Part model, mm, in its own coordinate system. A direction names the side the tool comes from. Give positions to 0.01 mm unless a question says otherwise; leave off trailing zeros. Order: outer loops, then holes, each group sorted by start corner. A loop starts at its lowest first (then second) coordinate and runs counter-clockwise, first axis right, second up. Notation, with made-up numbers: M 14.5,46.25 L 31.5,46.25 A14 ccw 31.5,53.25 Z; hole C -6,81 d2. An arc over 180 degrees is marked long. Answer as a JSON object with one key per item and string values.
from build123d import *

# Parameters (mm, degrees)
SKETCH1_W           = 30
SKETCH1_H           = 20
SKETCH1_H_2         = 2.5
SKETCH1_W_2         = 16
SKETCH1_W_3         = 7
SKETCH1_H_3         = 10.6
BOSS_EXTRUDE1_DEPTH = 6
SKETCH1_3_W         = 7
SKETCH1_3_H         = 2.5
SKETCH1_3_W_2       = 16
SKETCH1_3_W_3       = 30
BOSS_EXTRUDE2_DEPTH = 12
SKETCH3_R           = 1.5
CUT_EXTRUDE2_DEPTH  = 15
CUT_EXTRUDE1_DEPTH  = 38.976966704


with BuildPart() as part:
    # Sketch1 → Boss-Extrude1 (new body)
    with BuildSketch(Plane(origin=(0, 0, 0), x_dir=(1, 0, 0), z_dir=(0, 1, 0))):
        with Locations((-15, -10)):
            Rectangle(SKETCH1_W, SKETCH1_H)
        with Locations((-15, -21.25)):
            Rectangle(SKETCH1_W, SKETCH1_H_2)
        with Locations((-15, 1.25)):
            Rectangle(SKETCH1_W_2, SKETCH1_H_2)
        with Locations((-3.5, 1.25)):
            Rectangle(SKETCH1_W_3, SKETCH1_H_2)
        with Locations((-3.5, 7.8)):
            Rectangle(SKETCH1_W_3, SKETCH1_H_3)
        with Locations((-3.5, 14.35)):
            Rectangle(SKETCH1_W_3, SKETCH1_H_2)
        with Locations((-15, 14.35)):
            Rectangle(SKETCH1_W_2, SKETCH1_H_2)
        with Locations((-26.5, 14.35)):
            Rectangle(SKETCH1_W_3, SKETCH1_H_2)
        with Locations((-26.5, 7.8)):
            Rectangle(SKETCH1_W_3, SKETCH1_H_3)
        with Locations((-26.5, 1.25)):
            Rectangle(SKETCH1_W_3, SKETCH1_H_2)
    extrude(amount=BOSS_EXTRUDE1_DEPTH)

    # Sketch1_3 → Boss-Extrude2 (add)
    with BuildSketch(Plane(origin=(0, 0, 0), x_dir=(1, 0, 0), z_dir=(0, 1, 0))):
        with Locations((-3.5, 1.25)):
            Rectangle(SKETCH1_3_W, SKETCH1_3_H)
        with Locations((-15, 1.25)):
            Rectangle(SKETCH1_3_W_2, SKETCH1_3_H)
        with Locations((-15, -21.25)):
            Rectangle(SKETCH1_3_W_3, SKETCH1_3_H)
        with Locations((-26.5, 1.25)):
            Rectangle(SKETCH1_3_W, SKETCH1_3_H)
    extrude(amount=BOSS_EXTRUDE2_DEPTH)

    # Sketch3 → Cut-Extrude2 (cut)
    with BuildSketch(Plane(origin=(0, 0, -15.6), x_dir=(-1, 0, 0), z_dir=(0, 0, -1))):
        with Locations((15, 3)):
            Circle(SKETCH3_R)
    extrude(amount=-CUT_EXTRUDE2_DEPTH, mode=Mode.SUBTRACT)

    # Sketch2 → Cut-Extrude1 (cut, through all)
    with BuildSketch(Plane(origin=(0, 6, 0), x_dir=(1, 0, 0), z_dir=(0, 1, 0))):
        with BuildLine():
            ThreePointArc((-13, -10), (-15, -8), (-17, -10))
            Line((-17, -10), (-13, -10))
        make_face()
        with BuildLine():
            Line((-13, -10), (-17, -10))
            ThreePointArc((-17, -10), (-15, -12), (-13, -10))
        make_face()
    extrude(amount=-CUT_EXTRUDE1_DEPTH, mode=Mode.SUBTRACT)


solid = part.part
1. Probe line 1 along Z through (x, y) = (-20.5, 4); line 2 along Z through (x, y) = (-21.25, 9.5); line 3 along Z through (x, y) = (-15, 1.3). List the from-to ranges inside material, lowest first.
Worked answers:
{"line 1": "z = -15.6 to -13.1, -2.5 to 22.5", "line 2": "z = -2.5 to 0, 20 to 22.5", "line 3": "z = -15.6 to -13.1, -2.5 to 8, 12 to 22.5"}
2. Cut at C-C on z = 10. Give the cut face in (x, y).
Worked answers:
{"outline": "M -30,0 L -17,0 L -17,6 L -30,6 Z; M -13,0 L 0,0 L 0,6 L -13,6 Z"}
3. Cut at A-A on x = -20. Give the cut face in (y, z).
Worked answers:
{"outline": "M 0,-15.6 L 6,-15.6 L 6,-13.1 L 0,-13.1 Z; M 0,-2.5 L 12,-2.5 L 12,0 L 6,0 L 6,20 L 12,20 L 12,22.5 L 0,22.5 Z"}
4. Cut at B-B on y = 10. Give the cut face in (x, z).
Worked answers:
{"outline": "M -30,-2.5 L 0,-2.5 L 0,0 L -30,0 Z; M -30,20 L 0,20 L 0,22.5 L -30,22.5 Z"}
5. Two-plate mould, pull along Z, no slides. Class faces 1 (the cylindrical face through (-13.526, 3.042, 11.352)), 2 (the flat face through (-23, 3, -8)), 3 (the flat face through (-15, 6, 22.5)), 4 (the flat face through (-30, 5, 3)): +Z half, -Z half, draft (parallel to the pull), parting line (faces both ways), or undercut.
Worked answers:
{"face 1": "undercut", "face 2": "undercut", "face 3": "+Z half", "face 4": "draft"}
6. Which spindle directions (+Z, -Z, +X, -X, +Y, -Y) get a long thin tool onto all of the face, cutting with end or side? Do faces 5 (the flat face through (-7, 3, -8)), 6 (the flat face through (-15.2, 6, 7.6)), 7 (the flat face through (-15, 7, -2.5)), 8 (the flat face through (-15, 6, -14)), 9 (the cylindrical face through (-13.5, 3.07, -14.37)). Say none if no direction does.
Worked answers:
{"face 5": "+Y, -Y", "face 6": "+X, -X, +Y", "face 7": "+Y", "face 8": "-Z, +X, -X, +Y", "face 9": "-Z"}
7. Pin check, flat tips, straight feed: P1, Ø0.9, axis at x = -15.5, y = 3.5, coming from the -Z side; P2, Ø1, axis at x = -13.5, z = -11.5, coming from the -Y side; P3, Ø5, axis at x = -22, y = 10, coming from the -Z side; P4, Ø6.5, axis at x = -15, z = 10, coming from the +Y side. Stop position of each tip, or through.
Worked answers:
{"P1": "stops at z = -0.6", "P2": "passes through", "P3": "stops at z = -2.5", "P4": "stops at y = 6"}
8. Cut at D-D on y = 3. Give the cut face in (x, z).
Worked answers:
{"outline": "M -30,-15.6 L -16.5,-15.6 L -16.5,-13.1 L -23,-13.1 L -23,-2.5 L -16.5,-2.5 L -16.5,-0.6 L -13.5,-0.6 L -13.5,-2.5 L -7,-2.5 L -7,-13.1 L -13.5,-13.1 L -13.5,-15.6 L 0,-15.6 L 0,22.5 L -30,22.5 Z; hole C -15,10 d4"}
